```python
from build123d import *

# Parameters (mm, degrees)
SKETCH1_R           = 0.505
BOSS_EXTRUDE1_DEPTH = 1
CHAMFER1_SIZE       = 0.1
CHAMFER2_SIZE       = 0.1


with BuildPart() as part:
    # Sketch1 → Boss-Extrude1 (new, symmetric)
    with BuildSketch(Plane(origin=(0, 0, 0), x_dir=(1, 0, 0), z_dir=(0, 1, 0))):
        with BuildLine():
            ThreePointArc((-3.944558257, 1.11981448), (-5.61981448, 0.555441743), (-5.055441743, -1.11981448))
            ThreePointArc((-5.055441743, -1.11981448), (0, -2.304718782), (5.055441743, -1.11981448))
            ThreePointArc((5.055441743, -1.11981448), (5.61981448, 0.555441743), (3.944558257, 1.11981448))
            ThreePointArc((3.944558257, 1.11981448), (0, 0.195281218), (-3.944558257, 1.11981448))
        make_face()
        with Locations(Location((-4.5, 0, 0), (0, 0, 270))):
            Circle(SKETCH1_R, mode=Mode.SUBTRACT)
        with Locations(Location((4.5, 0, 0), (0, 0, 270))):
            Circle(SKETCH1_R, mode=Mode.SUBTRACT)
    extrude(amount=BOSS_EXTRUDE1_DEPTH, both=True)

    # Chamfer1
    chamfer1_edges = [part.edges().sort_by_distance(p)[0] for p in [
        (0, 1, 2.304718782),
        (5.61981448, 1, -0.555441743),
        (0, 1, -0.195281218),
        (5.61981448, -1, -0.555441743),
        (0, -1, 2.304718782),
        (-5.61981448, -1, -0.555441743),
        (0, -1, -0.195281218),
        (-5.61981448, 1, -0.555441743),
    ]]
    chamfer(chamfer1_edges, length=CHAMFER1_SIZE)

    # Chamfer2
    chamfer2_edges = [part.edges().sort_by_distance(p)[0] for p in [
        (-4.5, -1, -0.505),
        (-4.5, 1, -0.505),
        (4.5, -1, -0.505),
        (4.5, 1, -0.505),
    ]]
    chamfer(chamfer2_edges, length=CHAMFER2_SIZE)


solid = part.part
```
The listing builds one solid part. Answer for the finished solid, in the listing's coordinates (mm). Round coordinates to 2 decimals unless told otherwise and drop trailing zeros. Order: outer loops, then holes, each group sorted by start corner. A loop starts at its lowest first (then second) coordinate and runs counter-clockwise, first axis right, second up. Notation, with made-up numbers: (-30.75, -19) - (-19.75, -19) arc R18 cw to (-19.75, 11) - close; hole circle Ø6 at (43, 1). An arc over 180 degrees is marked (long way). Put each result on its own line as item: value. Start each with the question number.
(1) Straight lines are drawn through the part: probe 1 along X at (y, z) = (0.25, 0) (3 decimals); probe 2 along X at (y, z) = (0.5, 0.4); probe 3 along X at (y, z) = (0, -0.95). For each, find the intervals that lie inside material, in ascending order. Write a range as from..to.
(2) Given P1, Ø0.6, axis at x = 4.5, z = 0, coming from the +Y side, flat-ended and moving along its own axis, determine where the tip first touches the part or whether it passes through.
(3) Find section A-A (y = -0.2). Give the vertices of the cut face in (x, z) (3 decimals).
Reply:
1. probe 1: -5.75..-5.005, -3.995..3.995, 5.005..5.75
1. probe 2: -5.68..-4.81, -4.19..4.19, 4.81..5.68
1. probe 3: -5.31..-3.58, 3.58..5.31
2. P1: through
3. outline: (-5.055, 1.12) arc R1.25 ccw to (-3.945, -1.12) arc R8.877 cw to (3.945, -1.12) arc R1.25 ccw to (5.055, 1.12) arc R11.377 ccw to start; hole circle Ø1.01 at (-4.5, 0); hole circle Ø1.01 at (4.5, 0)
